Verification items for this drawing (mm, ordinates from the low corner). Give positions to 0.01 mm unless a question says otherwise; leave off trailing zeros. Order: outer loops, then holes, each group sorted by start corner. A loop starts at its lowest first (then second) coordinate and runs counter-clockwise, first axis right, second up. Notation, with made-up numbers: M 14.5,-31.5 L 58.5,-31.5 A27 ccw 58.5,-11.5 Z; hole C 33,20 d6. An arc over 180 degrees is marked long. Return JSON: item names as keys, results as strings. Group by question number.
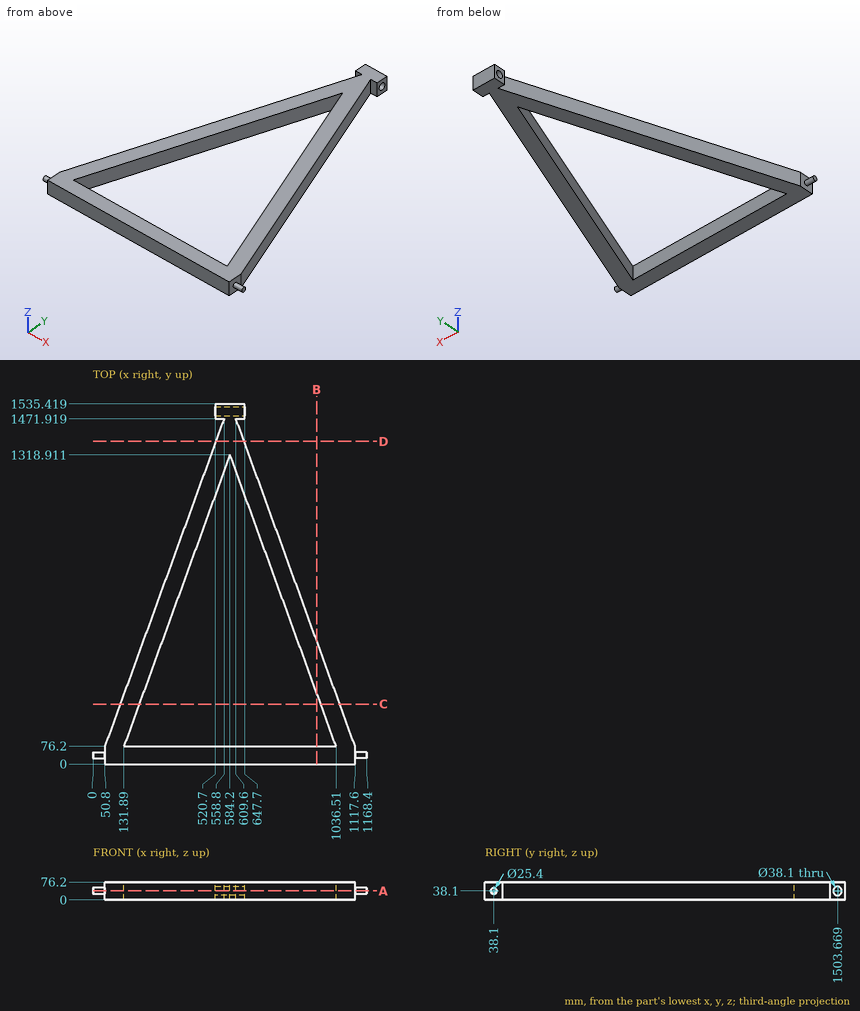
1) Sectioned sample at C-C on y = 255. Record the boundary of the cut face in (x, z).
2) Sectioned sample at A-A on z = 38.1. Record the boundary of the cut face in (x, y), then the cut area to 3 significant figures.
3) Depth check by flat-ended pin: P1, Ø3, axis at y = 1148.5, z = 15.5, coming from the +X side; P2, Ø19, axis at y = 1517, z = 46, coming from the -X side; P3, Ø3, axis at y = 299, z = 30.5, coming from the -X side; P4, Ø23, axis at y = 1503.67, z = 38.1, coming from the -X side. Enter the tip coordinate at first touch or a pass-through.
4) Material ranges on line 1 along X through (y, z) = (1191, 54.5) (1 decimal); line 2 along X through (y, z) = (1315.5, 46.5); line 3 along X through (y, z) = (1450, 32.5), recorded low to high.
5) Sectioned sample at B-B on x = 953.5. Record the boundary of the cut face in (y, z), then the cut area to 3 significant figures.
6) Sectioned sample at D-D on y = 1376.5. Record the boundary of the cut face in (x, z).
Reply:
{
 "1": {"outline": "M 115.88,0 L 196.97,0 L 196.97,76.2 L 115.88,76.2 Z; M 971.43,0 L 1052.52,0 L 1052.52,76.2 L 971.43,76.2 Z"},
 "2": {"outline": "M 0,25.4 L 50.8,25.4 L 50.8,0 L 1117.6,0 L 1117.6,25.4 L 1168.4,25.4 L 1168.4,50.8 L 1117.6,50.8 L 1117.6,76.2 L 609.6,1471.92 L 647.7,1471.92 L 647.7,1484.62 L 520.7,1484.62 L 520.7,1471.92 L 558.8,1471.92 L 50.8,76.2 L 50.8,50.8 L 0,50.8 Z; M 520.7,1522.72 L 647.7,1522.72 L 647.7,1535.42 L 520.7,1535.42 Z; hole M 131.89,76.2 L 1036.51,76.2 L 584.2,1318.91 Z", "area": "305,000 mm^2"},
 "3": {"P1": "x = 727.86", "P2": "x = 520.7", "P3": "x = 131.35", "P4": "through"},
 "4": {"line 1": "456.6 to 537.6, 630.8 to 711.8", "line 2": "501.87 to 582.96, 585.44 to 666.53", "line 3": "550.82 to 617.58"},
 "5": {"outline": "M 0,0 L 76.2,0 L 76.2,76.2 L 0,76.2 Z; M 304.27,0 L 527.06,0 L 527.06,76.2 L 304.27,76.2 Z", "area": "22,800 mm^2"},
 "6": {"outline": "M 524.07,0 L 644.33,0 L 644.33,76.2 L 524.07,76.2 Z"}
}
